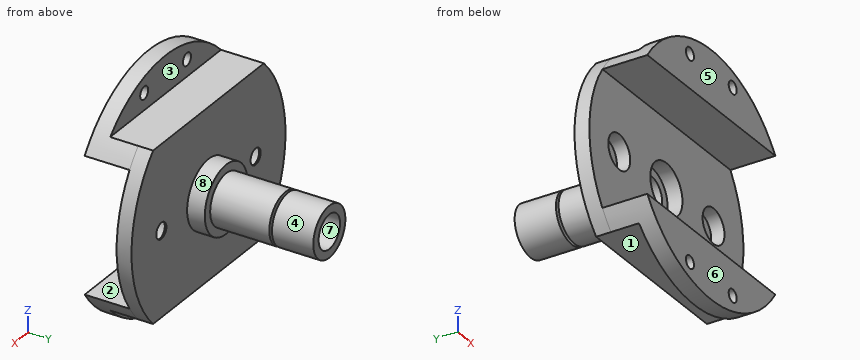
from build123d import *

# Parameters (mm, degrees)
SKETCH1_R           = 12.7
SKETCH1_R_2         = 6.35
BOSS_EXTRUDE1_DEPTH = 6.6548
SKETCH2_R           = 9.525
SKETCH2_R_2         = 6.35
BOSS_EXTRUDE2_DEPTH = 38.735
SKETCH3_OUTSIDE_W   = 38.976
SKETCH3_OUTSIDE_H   = 38.976
SKETCH3_OUTSIDE_R   = 7.4676
CUT_EXTRUDE1_DEPTH  = 0.9906
SKETCH5_R           = 45.72
SKETCH5_R_2         = 9.525
SKETCH5_R_3         = 3
BOSS_EXTRUDE4_DEPTH = 5.587499906
SKETCH6_R           = 6.5
CUT_EXTRUDE5_DEPTH  = 4.999999906
BOSS_EXTRUDE5_DEPTH = 16.875
SKETCH9_R           = 2.38125
CUT_EXTRUDE7_DEPTH  = 22.4625
SKETCH12_W          = 91.44
SKETCH12_H          = 13.97
CUT_EXTRUDE10_DEPTH = 16.1125


with BuildPart() as part:
    # Sketch1 → Boss-Extrude1 (new body)
    with BuildSketch(Plane(origin=(0, 0, 0), x_dir=(1, 0, 0), z_dir=(0, 1, 0))):
        Circle(SKETCH1_R)
        Circle(SKETCH1_R_2, mode=Mode.SUBTRACT)
    extrude(amount=BOSS_EXTRUDE1_DEPTH)

    # Sketch2 → Boss-Extrude2 (add)
    with BuildSketch(Plane(origin=(0, 6.6548, 0), x_dir=(1, 0, 0), z_dir=(0, 1, 0))):
        Circle(SKETCH2_R)
        Circle(SKETCH2_R_2, mode=Mode.SUBTRACT)
    extrude(amount=BOSS_EXTRUDE2_DEPTH)

    # Sketch3 outside → Cut-Extrude1 (cut)
    with BuildSketch(Plane(origin=(0, 28.8798, 0), x_dir=(-1, 0, 0), z_dir=(0, 1, 0))):
        Rectangle(SKETCH3_OUTSIDE_W, SKETCH3_OUTSIDE_H)
        Circle(SKETCH3_OUTSIDE_R, mode=Mode.SUBTRACT)
    extrude(amount=CUT_EXTRUDE1_DEPTH, mode=Mode.SUBTRACT)

    # Sketch5 → Boss-Extrude4 (add)
    with BuildSketch(Plane.XZ):
        Circle(SKETCH5_R)
        Circle(SKETCH5_R_2, mode=Mode.SUBTRACT)
        with Locations((28, 0)):
            Circle(SKETCH5_R_3, mode=Mode.SUBTRACT)
        with Locations((-28, 0)):
            Circle(SKETCH5_R_3, mode=Mode.SUBTRACT)
    extrude(amount=BOSS_EXTRUDE4_DEPTH)

    # Sketch6 → Cut-Extrude5 (cut)
    with BuildSketch(Plane.XZ.offset(5.587499906)):
        with Locations((-28, 0)):
            Circle(SKETCH6_R)
        with Locations((28, 0)):
            Circle(SKETCH6_R)
    extrude(amount=-CUT_EXTRUDE5_DEPTH, mode=Mode.SUBTRACT)

    # Sketch8 → Boss-Extrude5 (add)
    with BuildSketch(Plane.XZ.offset(5.587499906)):
        with BuildLine():
            Line((38.01523905, -25.4), (-38.01523905, -25.4))
            ThreePointArc((-38.01523905, -25.4), (0, -45.72), (38.01523905, -25.4))
        make_face()
        with BuildLine():
            ThreePointArc((38.01523905, 25.4), (0, 45.72), (-38.01523905, 25.4))
            Line((-38.01523905, 25.4), (38.01523905, 25.4))
        make_face()
    extrude(amount=BOSS_EXTRUDE5_DEPTH)

    # Sketch9 → Cut-Extrude7 (cut)
    with BuildSketch(Plane.XZ.offset(22.462499906)):
        with Locations((12.7, 38.1)):
            Circle(SKETCH9_R)
        with Locations((-12.7, 38.1)):
            Circle(SKETCH9_R)
        with Locations((-12.7, -38.1)):
            Circle(SKETCH9_R)
        with Locations((12.7, -38.1)):
            Circle(SKETCH9_R)
    extrude(amount=-CUT_EXTRUDE7_DEPTH, mode=Mode.SUBTRACT)

    # Sketch12 → Cut-Extrude10 (cut)
    with BuildSketch(Plane(origin=(0, 0, 0), x_dir=(1, 0, 0), z_dir=(0, 1, 0))):
        with Locations((0, -38.735)):
            Rectangle(SKETCH12_W, SKETCH12_H)
        with Locations((0, 38.735)):
            Rectangle(SKETCH12_W, SKETCH12_H)
    extrude(amount=-CUT_EXTRUDE10_DEPTH, mode=Mode.SUBTRACT)


solid = part.part
Geometry check sheet. Reference: the model listing, model coordinates, mm. Face numbers are marked on the shaded views. A direction names the side the tool comes from. Give positions to 0.01 mm unless a question says otherwise; leave off trailing zeros. Order: outer loops, then holes, each group sorted by start corner. A loop starts at its lowest first (then second) coordinate and runs counter-clockwise, first axis right, second up.
1) Cross-section at B-B (z = -38.1). Record the boundary of the cut face in (x, y), then the cut area to 3 significant figures.
Results are:
outline: (-25.27, -22.46) - (-15.08, -22.46) - (-15.08, -16.11) - (-25.27, -16.11) - close; (-10.32, -22.46) - (10.32, -22.46) - (10.32, -16.11) - (-10.32, -16.11) - close; (15.08, -22.46) - (25.27, -22.46) - (25.27, -16.11) - (15.08, -16.11) - close
area: 260 mm2
2) Tool access check on the marked faces 1, 2, 3, 4 and 5. Record the directions out of +Z, -Z, +X, -X, +Y, -Y that give a thin tool (end or side, any length) a straight path to the whole face; none if there is none.
Results are:
face 1: -Z, +X, -X, +Y
face 2: +X, -X, -Y
face 3: +Z, +X, -X, +Y
face 4: +Y
face 5: +Z, -Z, +X, -X, -Y
3) Draft check along X on the marked faces 6, 7 and 8. Enter one of: released by +X, released by -X, zero draft, split by the parting line, or undercut.
Results are:
face 6: zero draft
face 7: undercut
face 8: split by the parting line
4) Gauge pin test, flat ends, axial feed: pin 1 (6 mm diameter, centred on y = -4.5, z = -34, fed in from +X); pin 2 (7.5 mm diameter, centred on x = 12.7, z = -38.1, fed in from -Y); pin 3 (4 mm diameter, centred on x = -25, z = 0.5, fed in from -Y); pin 4 (8 mm diameter, centred on x = -9.5, y = -11, fed in from -Z). Record the tip position at first contact, or that the pin passes through.
Results are:
pin 1: stops at x = 33.61
pin 2: stops at y = -22.46
pin 3: stops at y = -0.59
pin 4: stops at z = -31.75
5) Cross-section at D-D (y = 33). Record the boundary of the cut face in (x, z) (3 decimals), then the cut area to 3 significant figures.
Results are:
outline: circle Ø19.05 at (0, 0); hole circle Ø12.7 at (0, 0)
area: 158 mm2
6) Material ranges on probe 1 along X at (y, z) = (-21, 38); probe 2 along Z at (x, y) = (0, 24.5) (3 decimals); probe 3 along Z at (x, y) = (0, -3) (3 decimals), recorded low to high.
Results are:
probe 1: x = -25.42 to -15.08, -10.32 to 10.32, 15.08 to 25.42
probe 2: z = -9.525 to -6.35, 6.35 to 9.525
probe 3: z = -31.75 to -9.525, 9.525 to 31.75
7) Cross-section at A-A (x = 28). Record the boundary of the cut face in (y, z), then the cut area to 3 significant figures.
Results are:
outline: (-22.46, -36.14) - (-16.11, -36.14) - (-16.11, -31.75) - (0, -31.75) - (0, -3) - (-0.59, -3) - (-0.59, -6.5) - (-5.59, -6.5) - (-5.59, -25.4) - (-22.46, -25.4) - close; (-22.46, 25.4) - (-5.59, 25.4) - (-5.59, 6.5) - (-0.59, 6.5) - (-0.59, 3) - (0, 3) - (0, 31.75) - (-16.11, 31.75) - (-16.11, 36.14) - (-22.46, 36.14) - close
area: 556 mm2
8) Cross-section at C-C (z = 0). Give the number of separate pieces and of enclosed holes in the cut face, then the cut area to 3 significant figures.
Results are:
separate pieces: 4
enclosed holes: 0
area: 594 mm2
